Part model, mm, in its own coordinate system. A direction names the side the tool comes from. Coordinates: 2 decimals unless noted, no trailing zeros. Order: outer loops, then holes, each group sorted by start corner. A loop starts at its lowest first (then second) coordinate and runs counter-clockwise, first axis right, second up.
from build123d import *

# Parameters (mm, degrees)
SKETCH1_R               = 12
SKETCH1_R_2             = 8
BOSS_EXTRUDE1_DEPTH     = 8
SKETCH1_3_R             = 8
BOSS_EXTRUDE2_DEPTH     = 115
CUT_EXTRUDE1_DEPTH      = 100
CUT_EXTRUDE1_DEPTH_BACK = 100
SKETCH3_R               = 2


with BuildPart() as part:
    # Sketch1 → Boss-Extrude1 (new body)
    # profile 1 of 2: a face of its own
    with BuildSketch(Plane.XY):
        Circle(SKETCH1_R)
        Circle(SKETCH1_R_2, mode=Mode.SUBTRACT)
    # profile 2 of 2: a face of its own
    with BuildSketch(Plane.XY):
        Circle(SKETCH1_R_2)
    extrude(amount=BOSS_EXTRUDE1_DEPTH)

    # Sketch1_3 → Boss-Extrude2 (add)
    with BuildSketch(Plane.XY):
        Circle(SKETCH1_3_R)
    extrude(amount=BOSS_EXTRUDE2_DEPTH)

    # Sketch3 → Cut-Extrude1 (cut, two sides: drawn at the far end of the back side and taken through both)
    with BuildSketch(Plane(origin=(0, 0, 0), x_dir=(0, 0, -1), z_dir=(1, 0, 0)).offset(-CUT_EXTRUDE1_DEPTH_BACK)):
        with Locations(Location((-102, 0, 0), (0, 0, 180))):
            Circle(SKETCH3_R)
    extrude(amount=CUT_EXTRUDE1_DEPTH + CUT_EXTRUDE1_DEPTH_BACK, mode=Mode.SUBTRACT)


solid = part.part
Q1. Mould opens along Y. For faces 1 (the face through (-11.99, 0.53, 3.94)), 2 (the face through (0, 0, 0)), 3 (the face through (-0.112, -0.601, 103.908)) say: pulls with the +Y half, pulls with the -Y half, needs draft (parallel to the pull), parting line crosses it, or undercut.
Results list:
face 1: parting line crosses it
face 2: needs draft
face 3: undercut
Q2. Cut at C-C on z = 26. Write the cut outline in (x, y), and give its area (3 significant figures).
Results list:
outline: circle Ø16 at (0, 0)
area: 201 mm2
Q3. Cut at B-B on x = 0. Write the cut outline in (y, z).
Results list:
outline: (-12, 0) - (12, 0) - (12, 8) - (8, 8) - (8, 115) - (-8, 115) - (-8, 8) - (-12, 8) - close; hole circle Ø4 at (0, 102)
Q4. Wall check: line 1 along Z through (x, y) = (-4.75, 7.25); line 2 along Y through (x, z) = (-0.5, 93); line 3 along Y through (x, z) = (2.5, 102). Give the ranges that are in metal, low to high.
Results list:
line 1: z = 0 to 8
line 2: y = -7.98 to 7.98
line 3: y = -7.6 to -2, 2 to 7.6
Q5. Which spindle directions (+Z, -Z, +X, -X, +Y, -Y) get a long thin tool onto all of the face, cutting with end or side? Do faces 4 (the face through (0, 0, 115)), 5 (the face through (-1.73, -7.81, 60.75)). Say none if no direction does.
Results list:
face 4: +Z, +X, -X, +Y, -Y
face 5: +Z
Q6. Cut at D-D on y = -7. Write the cut outline in (x, z).
Results list:
outline: (-9.75, 0) - (9.75, 0) - (9.75, 8) - (3.87, 8) - (3.87, 115) - (-3.87, 115) - (-3.87, 8) - (-9.75, 8) - close
Q7. Pin check, flat tips, straight feed: pin 1 Ø12 at (y, z) = (-8, 81) entering from -X; pin 2 Ø5 at (x, z) = (-3, 95.5) entering from +Y; pin 3 Ø2 at (y, z) = (8, 41) entering from +X. Stop position of each tip, or through.
Results list:
pin 1: stops at x = -7.75
pin 2: stops at y = 7.98
pin 3: stops at x = 3.87
Q8. Cut at A-A on y = 0. Write the cut outline in (x, z).
Results list:
outline: (-12, 0) - (12, 0) - (12, 8) - (8, 8) - (8, 100) - (-8, 100) - (-8, 8) - (-12, 8) - close; (-8, 104) - (8, 104) - (8, 115) - (-8, 115) - close
